Autodesk Inventor part; units mm, degrees
ref_plane "Work Plane1" through (0.377, 41.7467, 40.7) normal (0, 0, 1) x (1, 0, 0)
ref_plane "YZ Plane" through (0, 0, 0) normal (1, 0, 0) x (0, 1, 0)
ref_plane "XZ Plane" through (0, 0, 0) normal (0, 1, 0) x (-1, 0, 0)
sketch "Sketch1" plane through (0, 0, 0) normal (0, 0, 1) x (1, 0, 0)
  line L0 (-99.623, 141.7467) -> (100.377, 141.7467)
  line L1 (100.377, 141.7467) -> (100.377, -158.2533)
  line L2 (100.377, -158.2533) -> (-99.623, -158.2533)
  line L3 (-99.623, -158.2533) -> (-99.623, 141.7467)
  point P0 (0, 0)
  dimension "d0" = 200
  dimension "d1" = 300
extrude "Extrusion1" add sketch "Sketch1" along normal blind 10
sketch "Sketch2" plane through (0, 0, 10) normal (0, 0, 1) x (1, 0, 0)
  circle A0 centre (0.377, 41.7467) radius 50
  line L0 (100.377, 141.7467) -> (-99.623, 141.7467)
  line L1 (100.377, -158.2533) -> (100.377, 141.7467)
  point P0 (0, 0)
  dimension "d4" = 100
  dimension "d5" = 100
  dimension "d6" = 100
extrude "Extrusion2" add sketch "Sketch2" along normal blind 15
sketch "Sketch3" plane through (0.377, 41.7467, 25) normal (0, 0, 1) x (1, 0, 0)
  circle A0 centre (0, 0) radius 39.25
  point P0 (-0.377, -41.7467)
  dimension "d9" = 78.5
extrude "Extrusion3" add sketch "Sketch3" along normal blind 11.7
sketch "Sketch4" plane through (0.377, 41.7467, 36.7) normal (0, 0, 1) x (1, 0, 0)
  circle A0 centre (0, 0) radius 18.555
  point P0 (-0.377, -41.7467)
  dimension "d12" = 37.11
extrude "Extrusion4" add sketch "Sketch4" along normal blind 79
ref_plane "Work Plane1" through (0.377, 41.7467, 40.7) normal (0, 0, 1) x (1, 0, 0)
sketch "Sketch5" plane through (0.377, 41.7467, 40.7) normal (0, 0, 1) x (1, 0, 0)
  circle A0 centre (0, 0) radius 18.555
  circle A1 centre (0, 0) radius 29.09
  circle A2 centre (0, 0) radius 26.79
  line L0 (0, 0) -> (12.9512, 26.0479)
  line L1 (0, 0) -> (18.044, 22.8176)
  line L2 (0, 0) -> (-26.0479, 12.9512)
  line L3 (0, 0) -> (-22.8176, 18.044)
  line L4 (0, 0) -> (-12.9512, -26.0479)
  line L5 (0, 0) -> (-18.044, -22.8176)
  line L6 (0, 0) -> (26.0479, -12.9512)
  line L7 (0, 0) -> (22.8176, -18.044)
  point P0 (-0.377, -41.7467)
  point P1 (-23.9885, 11.9272)
  point P2 (-18.044, -22.8176)
  point P3 (-16.6174, -21.0135)
  point P4 (-11.9272, -23.9885)
  point P5 (22.8176, -18.044)
  point P6 (21.0135, -16.6174)
  point P7 (23.9885, -11.9272)
  point P8 (26.0479, -12.9512)
  point P9 (16.6174, 21.0135)
  point P10 (11.9272, 23.9885)
  point P11 (-21.0135, 16.6174)
  dimension "d16" = 58.18
  dimension "d19" = 53.58
  dimension "d20" = 11.9
  dimension "d23" = 360
extrude "Extrusion5" add sketch "Sketch5" along normal blind 15 contours A0 L1 A2 L6 | A0 L0 A2 L1 | L6 A2 L7 A0 | A0 L3 A2 L0 | L1 A1 L6 A2 | L7 A2 L4 A0 | A0 L2 A2 L3 | A2 L3 A1 L0 | A0 L5 A2 L2 | L4 A2 L5 A0 | L7 A1 L4 A2 | A2 L5 A1 L2
sketch "Sketch6" plane through (0.377, 41.7467, 115.7) normal (0, 0, 1) x (1, 0, 0)
  circle A0 centre (0, 0) radius 14
  point P0 (-0.377, -41.7467)
  dimension "d25" = 28
extrude "Extrusion6" cut sketch "Sketch6" against normal through all
sketch "Sketch7" plane through (0.377, 41.7467, 55.7) normal (0, 0, 1) x (1, 0, 0)
  circle A0 centre (0, 0) radius 14
  circle A1 centre (0, 0) radius 20
  point P0 (-0.377, -41.7467)
  dimension "d28" = 40
extrude "Extrusion7" add sketch "Sketch7" along normal blind 23.5
thread "Thread1"
properties part number "lathe_spindle_end"
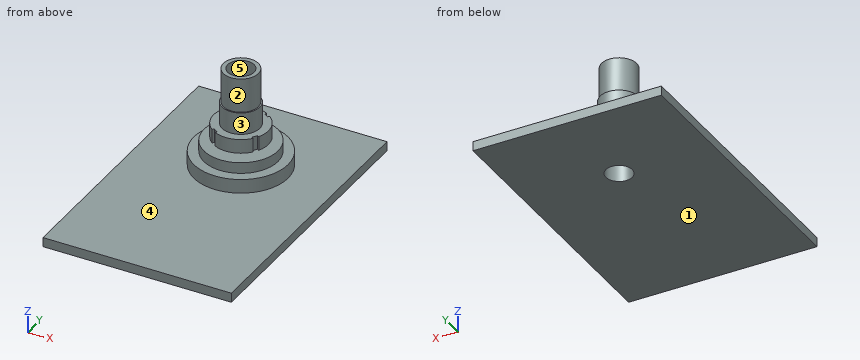
Could you check a few things on this model? Use its own coordinates, in mm. Face numbers are marked on the shaded views. A direction names the side the tool comes from. Give positions to 0.01 mm unless a question says otherwise; leave off trailing zeros. Write each loop counter-clockwise with the first axis right and the second up, starting at its lowest first coordinate (ties: lowest second). Pieces come first, ordered by that corner, then holes. Notation, with made-up numbers: (-3, 40) -> (28, 40) arc R22 cw to (28, 56) -> close; hole circle Ø7 at (-12.75, 17). An arc over 180 degrees is marked (long way). Write each question's results on one line, items separated by ' | '. Start each with the question number.
Q1. Suppose I cut it at A-A, the plane z = 51.5. List the corners of the cut face in (x, y) for me.
Q2. I need wall thicknesses on probe 1 along Z at (x, y) = (-9, 60.5); probe 2 along Z at (x, y) = (-88, -90.5); probe 3 along Z at (x, y) = (24, 63). Which ranges of each line are inside material? Lowest first, please.
Q3. Which directions (+Z, -Z, +X, -X, +Y, -Y) give clear straight access to the entire face, cutting with the end or side of a thin tool? Please do the marked faces 1 and 2.
Q4. Suppose I cut it at C-C, the plane y = -120. List the corners of the cut face in (x, z) for me.
Q5. We'd pull the mould along X, two halves only. Please class the marked faces 3, 4 and 5: +X half, -X half, draft (parallel to the pull), parting line (faces both ways), or undercut.
Q6. Suppose I cut it at D-D, the plane x = -65.5. List the corners of the cut face in (y, z) for me, and give its area (3 significant figures).
Q7. I'm going to push flat-ended pins straight in: pin 1 Ø8 at (x, y) = (35.5, 100.5) entering from +Z; pin 2 Ø5 at (x, z) = (16.5, 47.5) entering from -Y; pin 3 Ø4 at (x, z) = (-7, 88) entering from -Y; pin 4 Ø25 at (x, y) = (0.38, 41.75) entering from +Z. Where does each tip first touch, or does it pass through?
Outcome:
1) outline: (-25.67, 54.7) arc R29.09 ccw to (-17.67, 18.93) -> (-16.24, 20.73) arc R26.79 ccw to (-11.55, 17.76) -> (-12.57, 15.7) arc R29.09 ccw to (23.19, 23.7) -> (21.39, 25.13) arc R26.79 ccw to (24.37, 29.82) -> (26.42, 28.8) arc R29.09 ccw to (18.42, 64.56) -> (16.99, 62.76) arc R26.79 ccw to (12.3, 65.74) -> (13.33, 67.79) arc R29.09 ccw to (-22.44, 59.79) -> (-20.64, 58.36) arc R26.79 ccw to (-23.61, 53.67) -> close; hole circle Ø28 at (0.38, 41.75)
2) probe 1: 0 to 36.7, 40.7 to 55.7 | probe 2: 0 to 10 | probe 3: 0 to 36.7
3) face 1: -Z, +X, -X, +Y, -Y | face 2: +Z
4) outline: (-99.62, 0) -> (100.38, 0) -> (100.38, 10) -> (-99.62, 10) -> close
5) face 3: parting line | face 4: draft | face 5: undercut
6) outline: (-158.25, 0) -> (141.75, 0) -> (141.75, 10) -> (-158.25, 10) -> close | area: 3,000 mm2
7) pin 1: z = 10 | pin 2: y = 16.04 | pin 3: y = 23.99 | pin 4: through
